Model file for the job. Use its own axes, mm. Round coordinates to 2 decimals unless told otherwise and drop trailing zeros.
from build123d import *

# Parameters (mm, degrees)
SKETCH_1_R          = 1.25
SKETCH_1_R_2        = 1.5
EXTRUDE_1_DEPTH     = 2
CUT_EXTRUDE_1_DEPTH = 99.815339485


with BuildPart() as part:
    # 草图1 → 凸台-拉伸1 (new body)
    with BuildSketch(Plane(origin=(0, 0, 0), x_dir=(1, 0, 0), z_dir=(0, 1, 0))):
        with BuildLine():
            Line((-33, -81), (33, -81))
            ThreePointArc((33, -81), (38.656854249, -78.656854249), (41, -73))
            Line((41, -73), (41, 50.44414093))
            ThreePointArc((41, 50.44414093), (40.344059864, 53.616645416), (38.483803821, 56.268906647))
            Line((38.483803821, 56.268906647), (4.798328343, 87.982549413))
            ThreePointArc((4.798328343, 87.982549413), (0, 89.885879411), (-4.798328343, 87.982549413))
            Line((-4.798328343, 87.982549413), (-38.483803821, 56.268906647))
            ThreePointArc((-38.483803821, 56.268906647), (-40.344059864, 53.616645416), (-41, 50.44414093))
            Line((-41, 50.44414093), (-41, -73))
            ThreePointArc((-41, -73), (-38.656854249, -78.656854249), (-33, -81))
        make_face()
        with Locations(Location((-20, 30, 0), (0, 0, 270))):
            Circle(SKETCH_1_R, mode=Mode.SUBTRACT)
        with Locations(Location((20, 30, 0), (0, 0, 270))):
            Circle(SKETCH_1_R, mode=Mode.SUBTRACT)
        with Locations(Location((20, -30, 0), (0, 0, 270))):
            Circle(SKETCH_1_R, mode=Mode.SUBTRACT)
        with Locations(Location((-20, -30, 0), (0, 0, 270))):
            Circle(SKETCH_1_R, mode=Mode.SUBTRACT)
        with Locations(Location((0, 85.5, 0), (0, 0, 270))):
            Circle(SKETCH_1_R_2, mode=Mode.SUBTRACT)
        with Locations(Location((-36, 44, 0), (0, 0, 270))):
            Circle(SKETCH_1_R_2, mode=Mode.SUBTRACT)
        with Locations(Location((36, 44, 0), (0, 0, 270))):
            Circle(SKETCH_1_R_2, mode=Mode.SUBTRACT)
        with Locations(Location((36, -44, 0), (0, 0, 270))):
            Circle(SKETCH_1_R_2, mode=Mode.SUBTRACT)
        with Locations(Location((-36, -44, 0), (0, 0, 270))):
            Circle(SKETCH_1_R_2, mode=Mode.SUBTRACT)
        with Locations(Location((-32.5, 5, 0), (0, 0, 270))):
            Circle(SKETCH_1_R_2, mode=Mode.SUBTRACT)
        with Locations(Location((-32.5, -5, 0), (0, 0, 270))):
            Circle(SKETCH_1_R_2, mode=Mode.SUBTRACT)
        with Locations(Location((32.5, 5, 0), (0, 0, 270))):
            Circle(SKETCH_1_R_2, mode=Mode.SUBTRACT)
        with Locations(Location((32.5, -5, 0), (0, 0, 270))):
            Circle(SKETCH_1_R_2, mode=Mode.SUBTRACT)
        with Locations(Location((22.5, 0, 0), (0, 0, 270))):
            Circle(SKETCH_1_R_2, mode=Mode.SUBTRACT)
        with Locations(Location((-22.5, 0, 0), (0, 0, 270))):
            Circle(SKETCH_1_R_2, mode=Mode.SUBTRACT)
        with Locations(Location((-32.5, -63, 0), (0, 0, 270))):
            Circle(SKETCH_1_R_2, mode=Mode.SUBTRACT)
        with Locations(Location((-32.5, -73, 0), (0, 0, 270))):
            Circle(SKETCH_1_R_2, mode=Mode.SUBTRACT)
        with Locations(Location((-22.5, -68, 0), (0, 0, 270))):
            Circle(SKETCH_1_R_2, mode=Mode.SUBTRACT)
        with Locations(Location((32.5, -63, 0), (0, 0, 270))):
            Circle(SKETCH_1_R_2, mode=Mode.SUBTRACT)
        with Locations(Location((22.5, -68, 0), (0, 0, 270))):
            Circle(SKETCH_1_R_2, mode=Mode.SUBTRACT)
        with Locations(Location((32.5, -73, 0), (0, 0, 270))):
            Circle(SKETCH_1_R_2, mode=Mode.SUBTRACT)
        with Locations(Location((-18, 24, 0), (0, 0, 270))):
            Circle(SKETCH_1_R_2, mode=Mode.SUBTRACT)
        with Locations(Location((18, 24, 0), (0, 0, 270))):
            Circle(SKETCH_1_R_2, mode=Mode.SUBTRACT)
        with Locations(Location((18, -24, 0), (0, 0, 270))):
            Circle(SKETCH_1_R_2, mode=Mode.SUBTRACT)
        with Locations(Location((-18, -24, 0), (0, 0, 270))):
            Circle(SKETCH_1_R_2, mode=Mode.SUBTRACT)
        with Locations(Location((-28, 37, 0), (0, 0, 270))):
            Circle(SKETCH_1_R_2, mode=Mode.SUBTRACT)
        with Locations(Location((28, 37, 0), (0, 0, 270))):
            Circle(SKETCH_1_R_2, mode=Mode.SUBTRACT)
        with Locations(Location((-28, -37, 0), (0, 0, 270))):
            Circle(SKETCH_1_R_2, mode=Mode.SUBTRACT)
        with Locations(Location((28, -37, 0), (0, 0, 270))):
            Circle(SKETCH_1_R_2, mode=Mode.SUBTRACT)
        with BuildLine():
            Line((-37, 11), (-37, 36))
            ThreePointArc((-37, 36), (-35, 38), (-33, 36))
            Line((-33, 36), (-33, 11))
            ThreePointArc((-33, 11), (-35, 9), (-37, 11))
        make_face(mode=Mode.SUBTRACT)
        with BuildLine():
            Line((33, 11), (33, 36))
            ThreePointArc((33, 36), (35, 38), (37, 36))
            Line((37, 36), (37, 11))
            ThreePointArc((37, 11), (35, 9), (33, 11))
        make_face(mode=Mode.SUBTRACT)
        with BuildLine():
            Line((33, -36), (33, -11))
            ThreePointArc((33, -11), (35, -9), (37, -11))
            Line((37, -11), (37, -36))
            ThreePointArc((37, -36), (35, -38), (33, -36))
        make_face(mode=Mode.SUBTRACT)
        with BuildLine():
            Line((-37, -36), (-37, -11))
            ThreePointArc((-37, -11), (-35, -9), (-33, -11))
            Line((-33, -11), (-33, -36))
            ThreePointArc((-33, -36), (-35, -38), (-37, -36))
        make_face(mode=Mode.SUBTRACT)
    extrude(amount=EXTRUDE_1_DEPTH)

    # 草图3 → 切除-拉伸1 (cut, through all)
    with BuildSketch(Plane(origin=(0, 2, 0), x_dir=(1, 0, 0), z_dir=(0, 1, 0))):
        with BuildLine():
            Line((-22.0566638, 55), (-8, 55))
            ThreePointArc((-8, 55), (-5.878679656, 55.878679656), (-5, 58))
            Line((-5, 58), (-5, 71.233834699))
            ThreePointArc((-5, 71.233834699), (-6.810310818, 73.987857148), (-10.056426433, 73.418121843))
            Line((-10.056426433, 73.418121843), (-24.113090232, 60.184287144))
            ThreePointArc((-24.113090232, 60.184287144), (-24.845289037, 56.893849339), (-22.0566638, 55))
        make_face()
        with BuildLine():
            Line((22.0566638, 55), (8, 55))
            ThreePointArc((8, 55), (5.878679656, 55.878679656), (5, 58))
            Line((5, 58), (5, 71.233834699))
            ThreePointArc((5, 71.233834699), (6.810310818, 73.987857148), (10.056426433, 73.418121843))
            Line((10.056426433, 73.418121843), (24.113090232, 60.184287144))
            ThreePointArc((24.113090232, 60.184287144), (24.845289037, 56.893849339), (22.0566638, 55))
        make_face()
        Polygon((6.92820323, 12), (-6.92820323, 12), (-13.856406461, 0), (-6.92820323, -12), (6.92820323, -12), (13.856406461, 0), align=None)
        Polygon((13.856406461, 36), (6.92820323, 48), (-6.92820323, 48), (-13.856406461, 36), (-6.92820323, 24), (6.92820323, 24), align=None)
        Polygon((13.856406461, -36), (6.92820323, -24), (-6.92820323, -24), (-13.856406461, -36), (-6.92820323, -48), (6.92820323, -48), align=None)
        with BuildLine():
            Line((-14, -70.5), (14, -70.5))
            ThreePointArc((14, -70.5), (16.5, -73), (14, -75.5))
            Line((14, -75.5), (-14, -75.5))
            ThreePointArc((-14, -75.5), (-16.5, -73), (-14, -70.5))
        make_face()
        with BuildLine():
            Line((-18, -56.5), (18, -56.5))
            ThreePointArc((18, -56.5), (20.5, -59), (18, -61.5))
            Line((18, -61.5), (-18, -61.5))
            ThreePointArc((-18, -61.5), (-20.5, -59), (-18, -56.5))
        make_face()
    extrude(amount=-CUT_EXTRUDE_1_DEPTH, mode=Mode.SUBTRACT)


solid = part.part
Q1. Flat gauge pins, fed straight in: P1, Ø2.5, axis at x = 22.5, z = 0, coming from the +Y side; P2, Ø0.6, axis at x = 6, y = 1.5, coming from the -Z side; P3, Ø1, axis at y = 1.5, z = -70.5, coming from the -X side. Where does each tip first touch, or does it go through?
Q2. Slice it at A-A on y = 1.3. State how many separate pieces and enclosed holes the cut face has, plus the area to 3 significant figures.
Q3. Pull direction Z, two halves, no side cores. Call faces 1 (the face through (19.01, 0.99, 22.89)), 2 (the face through (21.88, 0.99, -71.9)): pulls with the +Z half, pulls with the -Z half, needs draft (parallel to the pull), parting line crosses it, or undercut.
Q4. Probe line 1 (X direction, y = 0.65, z = 20); line 2 (X direction, y = 0.95, z = 73); line 3 (X direction, y = 0.6, z = 5). List the from-to ranges inside material, lowest first.
Reply:
1. P1: passes through
1. P2: stops at z = -87.13
1. P3: stops at x = -23.9
2. separate pieces: 1
2. enclosed holes: 40
2. area: 9,580 mm2
3. face 1: undercut
3. face 2: pulls with the -Z half
4. line 1: x = -41 to -37, -33 to 33, 37 to 41
4. line 2: x = -41 to -34, -31 to -16.5, 16.5 to 31, 34 to 41
4. line 3: x = -41 to -34, -31 to -10.97, 10.97 to 31, 34 to 41
